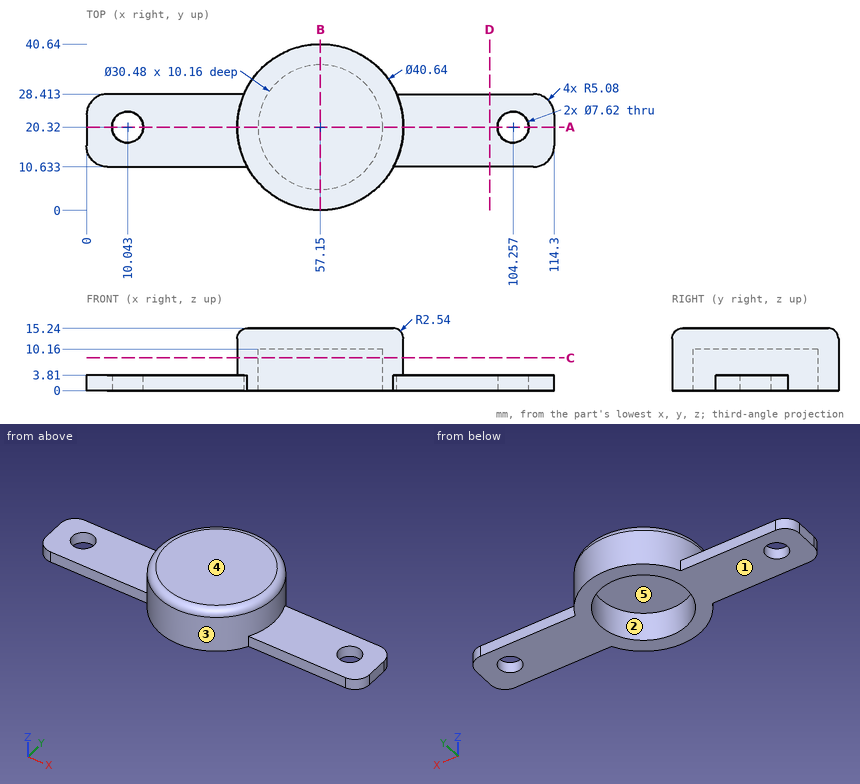
Study the drawing (mm; zero at the part's minimum x, y, z) and answer. A direction names the side the tool comes from. Coordinates: 2 decimals unless noted, no trailing zeros. Loops run counter-clockwise (first coordinate to the right, second up) from the corner with the lowest first, then second, coordinate; pieces in that order, holes last. Notation, with made-up numbers: M 50.5,49.5 L 90.5,49.5 A25 cw 90.5,70.5 Z; hole C 71,-2 d9. An arc over 180 degrees is marked long. Answer as a JSON object with one key per item and string values. Group by question number.
Item 1: Section D-D (x = 98.5) is taken. Write down the section's boundary in (y, z).
Item 2: Each of these flat-tipped pins is pushed along its axis until it touches: P1, Ø1.9, axis at x = 19, z = 1.5, coming from the -Y side; P2, Ø3, axis at x = 88.5, z = 2.5, coming from the +Y side; P3, Ø5, axis at x = 65, z = 7.5, coming from the +Y side. Where does it stop, or does it pass through?
Item 3: Determine the mould class of the marked faces 3, 4 and 5 for opening direction X: +X half, -X half, draft (parallel to the pull), parting line (faces both ways), or undercut.
Item 4: Section B-B (x = 57.15) is taken. Write down the section's boundary in (y, z).
Item 5: Section C-C (z = 8) is taken. Write down the section's boundary in (x, y).
Item 6: Section A-A (y = 20.32) is taken. Write down the section's boundary in (x, z).
Item 7: Consider L1, parallel to Y at x = 99, z = 2.5; L2, parallel to X at y = 16, z = 2.5 (1 decimal); L3, parallel to Z at x = 30, y = 18.5. Determine where each line is inside the solid, lowest interval first.
Item 8: Which of the six approach directions +Z, -Z, +X, -X, +Y, -Y give full straight-line access (tool end or side, diameter ignored) to the marked faces 1 and 2?
Solved:
{
 "1": {"outline": "M 10.63,0 L 28.41,0 L 28.41,3.81 L 10.63,3.81 Z"},
 "2": {"P1": "stops at y = 10.63", "P2": "stops at y = 28.41", "P3": "stops at y = 39.92"},
 "3": {"face 3": "parting line", "face 4": "draft", "face 5": "undercut"},
 "4": {"outline": "M 0,0 L 5.08,0 L 5.08,10.16 L 35.56,10.16 L 35.56,0 L 40.64,0 L 40.64,12.7 A2.54 ccw 38.1,15.24 L 2.54,15.24 A2.54 ccw 0,12.7 Z"},
 "5": {"outline": "C 57.15,20.32 d40.64; hole C 57.15,20.32 d30.48"},
 "6": {"outline": "M 0,0 L 6.23,0 L 6.23,3.81 L 0,3.81 Z; M 13.85,0 L 41.91,0 L 41.91,10.16 L 72.39,10.16 L 72.39,0 L 100.45,0 L 100.45,3.81 L 77.47,3.81 L 77.47,12.7 A2.54 ccw 74.93,15.24 L 39.37,15.24 A2.54 ccw 36.83,12.7 L 36.83,3.81 L 13.85,3.81 Z; M 108.07,0 L 114.3,0 L 114.3,3.81 L 108.07,3.81 Z"},
 "7": {"L1": "y = 10.63 to 28.41", "L2": "x = 0 to 42.5, 71.8 to 114.3", "L3": "z = 0 to 3.81"},
 "8": {"face 1": "-Z, +X, -X, +Y, -Y", "face 2": "-Z"}
}
